The model under review builds one solid part; all positions refer to its coordinate system, in mm. A direction names the side the tool comes from. Round coordinates to 2 decimals unless told otherwise and drop trailing zeros. Order: outer loops, then holes, each group sorted by start corner. A loop starts at its lowest first (then second) coordinate and runs counter-clockwise, first axis right, second up.
```python
from build123d import *

# Parameters (mm, degrees)
BOSS_EXTRUDE1_DEPTH = 46
CUT_EXTRUDE1_DEPTH  = 3
SKETCH3_R           = 2.25
CUT_EXTRUDE2_DEPTH  = 46
FILLET1_R           = 3


with BuildPart() as part:
    # Sketch1 → Boss-Extrude1 (new body)
    with BuildSketch(Plane.XY):
        Polygon((0, 0), (0, 65), (3, 65), (3, 3), (37, 3), (37, 0), align=None)
    extrude(amount=BOSS_EXTRUDE1_DEPTH)

    # Sketch2 → Cut-Extrude1 (cut)
    with BuildSketch(Plane.ZY):
        Polygon((0, 65), (14, 65), (15, 65), (15, 40), (14, 40), (14, 0), (0, 0), align=None)
        with BuildLine():
            Line((42, 46.5), (46, 46.5))
            Line((46, 46.5), (46, 36.5))
            Line((46, 36.5), (42, 36.5))
            ThreePointArc((42, 36.5), (37, 41.5), (42, 46.5))
        make_face()
    extrude(amount=-CUT_EXTRUDE1_DEPTH, mode=Mode.SUBTRACT)

    # Sketch3 → Cut-Extrude2 (cut)
    with BuildSketch(Plane(origin=(3, 0, 0), x_dir=(0, 0, -1), z_dir=(1, 0, 0))):
        with Locations(Location((-37.5, 55, 0), (0, 0, 90))):
            Circle(SKETCH3_R)
        with Locations(Location((-22.5, 55, 0), (0, 0, 90))):
            Circle(SKETCH3_R)
    extrude(amount=-CUT_EXTRUDE2_DEPTH, mode=Mode.SUBTRACT)

    # Fillet1
    # the kernel refuses this fillet: 3 mm, written as the material it adds along each edge
    with BuildSketch(Plane(origin=(3, 3, 14), x_dir=(0, 1, 0), z_dir=(0, 0, 1))) as fillet1_piece_1:
        with BuildLine():
            CenterArc((FILLET1_R, -FILLET1_R), FILLET1_R, 90, 90)
            Line((0, -FILLET1_R), (0, 0))
            Line((0, 0), (FILLET1_R, 0))
        make_face()
    extrude(amount=32)
    # the kernel refuses this fillet: 3 mm, written as the material it takes off along each edge
    with BuildSketch(Plane(origin=(-5.590169944, 40, 14), x_dir=(0, -1, 0), z_dir=(1, 0, 0))) as fillet1_2_piece_1:
        with BuildLine():
            CenterArc((2.236067977, -3), FILLET1_R, 90, 48.189685104)
            Line((0, -1), (0, 0))
            Line((0, 0), (2.236067977, 0))
        make_face()
    extrude(amount=14.180339887, mode=Mode.SUBTRACT)
    with BuildSketch(Plane(origin=(37, 10.5, 46), x_dir=(-1, 0, 0), z_dir=(0, -1, 0)), Plane(origin=(3, -7.5, 0), x_dir=(0, 0, 1), z_dir=(0, 1, 0))) as fillet1_2_piece_2:
        with BuildLine():
            CenterArc((FILLET1_R, FILLET1_R), FILLET1_R, 180, 90)
            Line((0, FILLET1_R), (0, 0))
            Line((0, 0), (FILLET1_R, 0))
        make_face()
    extrude(amount=18, mode=Mode.SUBTRACT)
    with BuildSketch(Plane(origin=(37, 10.5, 0), x_dir=(-1, 0, 0), z_dir=(0, -1, 0)), Plane(origin=(-7.5, 65, 46), x_dir=(0, 0, -1), z_dir=(1, 0, 0)), Plane(origin=(-7.5, 65, 15), x_dir=(0, -1, 0), z_dir=(1, 0, 0))) as fillet1_2_piece_3:
        with BuildLine():
            CenterArc((FILLET1_R, -FILLET1_R), FILLET1_R, 90, 90)
            Line((0, -FILLET1_R), (0, 0))
            Line((0, 0), (FILLET1_R, 0))
        make_face()
    extrude(amount=18, mode=Mode.SUBTRACT)


solid = part.part
```
(1) Consider section C-C (y = 34.5). Write out the cut boundary in (x, z), and give its area (3 significant figures).
Data:
outline: (0, 14) - (3, 14) - (3, 46) - (0, 46) - close
area: 96.0 mm2
(2) Draft analysis for pull direction Y (two halves, no side actions). For faces 1 (the flat face through (1, 46.5, 44)), 2 (the flat face through (1, 36.5, 44)), 3 (the cylindrical face through (1.48, 64.14, 45.1)), 4 (the flat face through (3, 2, 9)), state which applies: pulls with the +Y half, pulls with the -Y half, needs draft (parallel to the pull), parting line crosses it, or undercut.
Data:
face 1: undercut
face 2: undercut
face 3: pulls with the +Y half
face 4: needs draft
(3) Consider section D-D (x = 32.5). Write out the cut boundary in (y, z), and give its area (3 significant figures).
Data:
outline: (0, 0) - (3, 0) - (3, 46) - (0, 46) - close
area: 138 mm2
(4) To check wall thickness, follow probe 1 along Z at (x, y) = (2.25, 55); probe 2 along Y at (x, z) = (20, 28). State the ranges of each line that lie inside material, in increasing order.
Data:
probe 1: z = 15 to 20.25, 24.75 to 35.25, 39.75 to 46
probe 2: y = 0 to 3
(5) Insertion check: pin 1 (16 mm diameter, centred on y = 39, z = 35, fed in from +X); pin 2 (2 mm diameter, centred on x = 9.5, z = 10.5, fed in from +Y); pin 3 (6 mm diameter, centred on y = 19, z = 24, fed in from -X); pin 4 (0.9 mm diameter, centred on x = 1.5, y = 55, fed in from -Z). Each pin has a flat end and moves straight along its axis. Give the tip position at first contact, or say it passes through.
Data:
pin 1: stops at x = 3
pin 2: stops at y = 3
pin 3: stops at x = 0
pin 4: stops at z = 15
(6) Consider section B-B (z = 22.5). Write out the cut boundary in (x, y).
Data:
outline: (0, 0) - (37, 0) - (37, 3) - (6, 3) arc R3 cw to (3, 6) - (3, 52.75) - (0, 52.75) - close; (0, 57.25) - (3, 57.25) - (3, 65) - (0, 65) - close
(7) Consider section A-A (y = 55). Write out the cut boundary in (x, z), and give its area (3 significant figures).
Data:
outline: (0, 15) - (3, 15) - (3, 20.25) - (0, 20.25) - close; (0, 24.75) - (3, 24.75) - (3, 35.25) - (0, 35.25) - close; (0, 39.75) - (3, 39.75) - (3, 46) - (0, 46) - close
area: 66.0 mm2
(8) For faces 5 (the flat face through (3, 36, 30)), 6 (the cylindrical face through (1.48, 64.1, 15.86)), list the 3-axis set-ups (+Z, -Z, +X, -X, +Y, -Y) from which the entire face can be reached by the end or side of a thin tool; tool diameter is ignored.
Data:
face 5: +Z, -Z, +X, +Y
face 6: -Z, +X, -X, +Y
